Read the model definition and answer for the solid it produces. Units are mm, in the model's axes. Face numbers are marked on the shaded views. A direction names the side the tool comes from. Coordinates: 2 decimals unless noted, no trailing zeros. Loops run counter-clockwise (first coordinate to the right, second up) from the corner with the lowest first, then second, coordinate; pieces in that order, holes last. Notation, with made-up numbers: (2.5, 56.25) -> (50.5, 56.25) arc R14 cw to (50.5, 81.25) -> close; hole circle Ø3 at (29, -39). An arc over 180 degrees is marked (long way). Answer in a Markdown table with one row per item.
```python
from build123d import *

# Parameters (mm, degrees)
F0_W     = 53.7313818932
F0_H     = 72.609975934
F1_DEPTH = 75.4805505276
F0_W_2   = 40.0392413139
F0_H_2   = 23.0277478695
F2_DEPTH = 30.2285254002
F3_DEPTH = 100.3713980317


with BuildPart() as f1:
    # F0 (on Front) → F1 (new body)
    with BuildSketch(Plane.XZ):
        with Locations((172.2931265831, 4.7715082765)):
            Rectangle(F0_W, F0_H)
        with BuildLine():
            ThreePointArc((199.1588175297, 41.0764962435), (225.7710662807, 124.9978706097), (145.4274356365, 88.9991223812))
            Line((145.4274356365, 88.9991223812), (145.4274356365, 41.0764962435))
            Line((145.4274356365, 41.0764962435), (199.1588175297, 41.0764962435))
        make_face()
        with BuildLine():
            Line((145.4274356365, -31.5334796906), (88.5841548443, -31.5334796906))
            Line((88.5841548443, -31.5334796906), (88.5841548443, -86.717069149))
            ThreePointArc((88.5841548443, -86.717069149), (160.9384717068, -93.3234153061), (199.1588175297, -31.5334796906))
            Line((199.1588175297, -31.5334796906), (145.4274356365, -31.5334796906))
        make_face()
    extrude(amount=F1_DEPTH)

    # F0 (on Front) → F2 (join)
    with BuildSketch(Plane.XZ):
        Polygon((128.6233961582, 88.9991223812), (88.5841548443, 88.9991223812), (88.5841548443, -31.5334796906), (145.4274356365, -31.5334796906), (145.4274356365, 41.0764962435), (145.4274356365, 88.9991223812), align=None)
        with Locations((108.6037755013, 100.512996316)):
            Rectangle(F0_W_2, F0_H_2)
        with BuildLine():
            Line((145.4274356365, -31.5334796906), (88.5841548443, -31.5334796906))
            Line((88.5841548443, -31.5334796906), (88.5841548443, -86.717069149))
            ThreePointArc((88.5841548443, -86.717069149), (160.9384717068, -93.3234153061), (199.1588175297, -31.5334796906))
            Line((199.1588175297, -31.5334796906), (145.4274356365, -31.5334796906))
        make_face()
        with BuildLine():
            ThreePointArc((199.1588175297, 41.0764962435), (225.7710662807, 124.9978706097), (145.4274356365, 88.9991223812))
            Line((145.4274356365, 88.9991223812), (145.4274356365, 41.0764962435))
            Line((145.4274356365, 41.0764962435), (199.1588175297, 41.0764962435))
        make_face()
        with Locations((172.2931265831, 4.7715082765)):
            Rectangle(F0_W, F0_H)
    extrude(amount=F2_DEPTH)

    # F0 (on Front) → F3 (join)
    with BuildSketch(Plane.XZ):
        Polygon((88.5841548443, -31.5334796906), (88.5841548443, 88.9991223812), (-88.5842293501, 88.9991223812), (-88.5842293501, -86.717069149), (88.5841548443, -86.717069149), align=None)
    extrude(amount=F3_DEPTH)


solid = f1.part
```
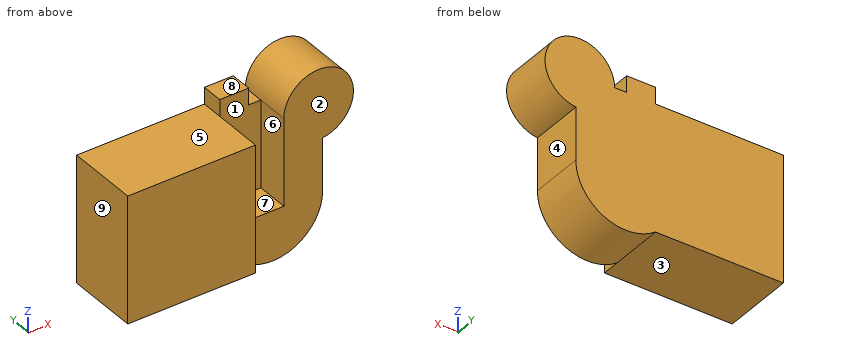
1. A tool of negligible diameter and unlimited length cuts with its end or side. For the marked faces 1, 2, 3, 4 and 5, from which of +Z, -Z, +X, -X, +Y, -Y can it reach the whole face along a straight path? Write none if from no direction.
A:
| item | result |
|---|---|
| face 1 | +Z, -Y |
| face 2 | +Z, -Z, +X, -Y |
| face 3 | -Z, -X, +Y, -Y |
| face 4 | -Z, +X, +Y, -Y |
| face 5 | +Z, -X, +Y, -Y |
2. Find the intervals of material crossed by probe 1 along X at (y, z) = (-47, -25); probe 2 along Z at (x, y) = (-45.5, -6.5); probe 3 along X at (y, z) = (-94, 48), in increasing order.
A:
| item | result |
|---|---|
| probe 1 | x = -88.58 to 88.58, 145.43 to 199.16 |
| probe 2 | z = -86.72 to 89 |
| probe 3 | x = -88.58 to 88.58 |
3. A cutting plane is placed at A-A on y = -37. Give the vertices of the cut face in (x, z), and give its area (3 significant figures).
A:
| item | result |
|---|---|
| outline | (-88.58, -86.72) -> (88.58, -86.72) arc R69.06 ccw to (199.16, -31.53) -> (199.16, 41.08) arc R48.24 ccw (long way) to (145.43, 89) -> (145.43, -31.53) -> (88.58, -31.53) -> (88.58, 89) -> (-88.58, 89) -> close |
| area | 49,300 mm2 |
4. Given pin 1 Ø6 at (y, z) = (-49, 57.5) entering from +X; pin 2 Ø2 at (x, y) = (25.5, -61) entering from +Z; pin 3 Ø21 at (y, z) = (-50, -10.5) entering from +X, each flat-ended and moving along its own axis, determine where each tip first touches the part or whether it passes through.
A:
| item | result |
|---|---|
| pin 1 | stops at x = 232.58 |
| pin 2 | stops at z = 89 |
| pin 3 | stops at x = 199.16 |
5. A cutting plane is placed at C-C on z = 23. Give the vertices of the cut face in (x, y).
A:
| item | result |
|---|---|
| outline | (-88.58, -100.37) -> (88.58, -100.37) -> (88.58, -30.23) -> (145.43, -30.23) -> (145.43, -75.48) -> (199.16, -75.48) -> (199.16, 0) -> (-88.58, 0) -> close |
6. A cutting plane is placed at B-B on z = 96. Give the vertices of the cut face in (x, y), and give its area (3 significant figures).
A:
| item | result |
|---|---|
| outline | (88.58, -30.23) -> (128.62, -30.23) -> (128.62, 0) -> (88.58, 0) -> close; (145.94, -75.48) -> (241.39, -75.48) -> (241.39, 0) -> (145.94, 0) -> close |
| area | 8,420 mm2 |
7. A cutting plane is placed at D-D on x = -34.5. Give the vertices of the cut face in (y, z), and give its area (3 significant figures).
A:
| item | result |
|---|---|
| outline | (-100.37, -86.72) -> (0, -86.72) -> (0, 89) -> (-100.37, 89) -> close |
| area | 17,600 mm2 |
8. The mould has two halves that part along X. Classify the marked faces 6, 7, 8 and 9: pulls with the +X half, pulls with the -X half, needs draft (parallel to the pull), parting line crosses it, or undercut.
A:
| item | result |
|---|---|
| face 6 | undercut |
| face 7 | undercut |
| face 8 | needs draft |
| face 9 | pulls with the -X half |
